from build123d import *

# Parameters (mm, degrees)
SALIENTE_EXTRUIR1_DEPTH = 5.75
CROQUIS2_W              = 25
CROQUIS2_H              = 25
SALIENTE_EXTRUIR2_DEPTH = 3
CROQUIS3_W              = 21.75
CROQUIS3_H              = 21.75
CROQUIS3_W_2            = 13.5
CROQUIS3_H_2            = 13.5
SALIENTE_EXTRUIR3_DEPTH = 13
CORTAR_EXTRUIR1_DEPTH   = 13
CORTAR_EXTRUIR2_DEPTH   = 13
SALIENTE_EXTRUIR4_DEPTH = 2


with BuildPart() as part:
    # Croquis1 → Saliente-Extruir1 (new, symmetric)
    with BuildSketch(Plane(origin=(0, 0, 0), x_dir=(1, 0, 0), z_dir=(0, 1, 0))):
        Polygon((0, 0), (15, 0), (15, -10), (-10, -10), (-10, 15), (0, 15), align=None)
    extrude(amount=SALIENTE_EXTRUIR1_DEPTH, both=True)

    # Croquis2 → Saliente-Extruir2 (add)
    with BuildSketch(Plane.XZ.offset(5.75)):
        with Locations((2.5, -2.5)):
            Rectangle(CROQUIS2_W, CROQUIS2_H)
    extrude(amount=SALIENTE_EXTRUIR2_DEPTH)

    # Croquis3 → Saliente-Extruir3 (add)
    with BuildSketch(Plane.XZ.offset(8.75)):
        with Locations((0.875, -0.875)):
            Rectangle(CROQUIS3_W, CROQUIS3_H)
        with Locations((2.5, -2.5)):
            Rectangle(CROQUIS3_W_2, CROQUIS3_H_2, mode=Mode.SUBTRACT)
    extrude(amount=SALIENTE_EXTRUIR3_DEPTH)

    # Croquis4 → Cortar-Extruir1 (cut)
    with BuildSketch(Plane(origin=(11.75, 0, 0), x_dir=(0, 0, -1), z_dir=(1, 0, 0))):
        with BuildLine():
            Line((-1.125, -12.25), (-1.125, -18.25))
            ThreePointArc((-1.125, -18.25), (0.875, -20.25), (2.875, -18.25))
            Line((2.875, -18.25), (2.875, -12.25))
            ThreePointArc((2.875, -12.25), (0.875, -10.25), (-1.125, -12.25))
        make_face()
    extrude(amount=-CORTAR_EXTRUIR1_DEPTH, mode=Mode.SUBTRACT)

    # Croquis6 → Cortar-Extruir2 (cut)
    with BuildSketch(Plane(origin=(0, 0, -11.75), x_dir=(-1, 0, 0), z_dir=(0, 0, -1))):
        with BuildLine():
            Line((1.125, -12.25), (1.125, -18.25))
            ThreePointArc((1.125, -18.25), (-0.875, -20.25), (-2.875, -18.25))
            Line((-2.875, -18.25), (-2.875, -12.25))
            ThreePointArc((-2.875, -12.25), (-0.875, -10.25), (1.125, -12.25))
        make_face()
    extrude(amount=-CORTAR_EXTRUIR2_DEPTH, mode=Mode.SUBTRACT)

    # Croquis7 → Saliente-Extruir4 (add)
    with BuildSketch(Plane(origin=(0, 5.75, 0), x_dir=(1, 0, 0), z_dir=(0, 1, 0))):
        Polygon((15, 0), (0, 15), (0, 0), align=None)
        Polygon((15, 0), (0, 0), (0, 15), (-10, 15), (-10, -10), (15, -10), align=None)
    extrude(amount=SALIENTE_EXTRUIR4_DEPTH)


solid = part.part
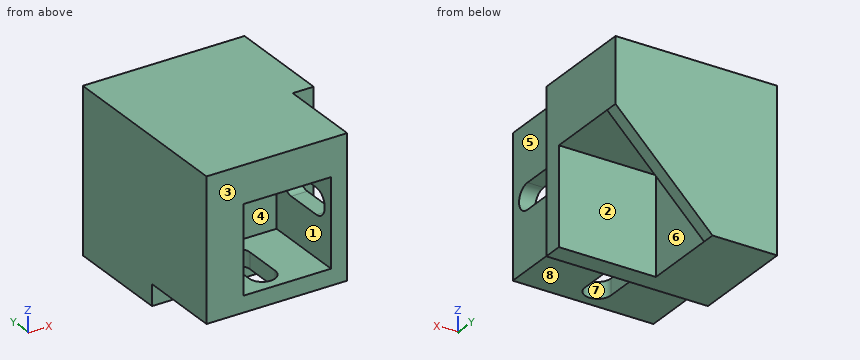
CAD build for the part. Positions are in the model's coordinates, mm. Face numbers are marked on the shaded views. A direction names the side the tool comes from. Coordinates: 2 decimals unless noted, no trailing zeros. Write each loop counter-clockwise with the first axis right and the second up, starting at its lowest first coordinate (ties: lowest second). Pieces come first, ordered by that corner, then holes. Notation, with made-up numbers: M 66.5,8 L 99.5,8 A25 ccw 99.5,27 Z; hole C 25,8 d10. An arc over 180 degrees is marked long. Return JSON: item names as keys, results as strings.
Item 1: Drop flat-ended pins along their axis: pin 1 Ø6.5 at (y, z) = (-12.5, -2) entering from +X; pin 2 Ø3 at (x, y) = (11, -14.5) entering from -Z; pin 3 Ø4 at (x, z) = (3.5, 0.5) entering from -Y. Give the stop position or say it passes through.
Findings below:
{"pin 1": "stops at x = 11.75", "pin 2": "stops at z = -11.75", "pin 3": "stops at y = -8.75"}
Item 2: Slice it at B-B, the plane y = -16.75. Write the cut outline in (x, z) (3 decimals).
Findings below:
{"outline": "M -10,-11.75 L -1.125,-11.75 L -1.125,-9.25 L -4.25,-9.25 L -4.25,4.25 L 9.25,4.25 L 9.25,1.125 L 11.75,1.125 L 11.75,10 L -10,10 Z; M 2.875,-11.75 L 11.75,-11.75 L 11.75,-2.875 L 9.25,-2.875 L 9.25,-9.25 L 2.875,-9.25 Z"}
Item 3: Which spindle directions (+Z, -Z, +X, -X, +Y, -Y) get a long thin tool onto all of the face, cutting with end or side? Do the marked faces 4, 5, 6, 7 and 8. Say none if no direction does.
Findings below:
{"face 4": "-Y", "face 5": "+Z, -Z, +X, -Y", "face 6": "-Z, +X", "face 7": "-Z", "face 8": "-Z, +X, -X, -Y"}
Item 4: Slice it at D-D, the plane z = -0.5. Write the cut outline in (x, y), and give its area (3 significant figures).
Findings below:
{"outline": "M -10,-21.75 L -4.25,-21.75 L -4.25,-8.75 L 9.25,-8.75 L 9.25,-10.29 L 11.75,-10.29 L 11.75,-8.75 L 15,-8.75 L 15,-5.75 L 0,-5.75 L 0,5.75 L 14.5,5.75 L 14.5,7.75 L -10,7.75 Z; M 9.25,-21.75 L 11.75,-21.75 L 11.75,-20.21 L 9.25,-20.21 Z", "area": "321 mm2"}
Item 5: Probe line 1 (X direction, y = -18.5, z = -4); line 2 (Y direction, x = 3.5, z = -2); line 3 (Z direction, x = 7.75, y = -16.75). List the from-to ranges inside material, lowest first. Write a range as from..to.
Findings below:
{"line 1": "x = -10..-4.25, 9.25..11.75", "line 2": "y = -8.75..-5.75, 5.75..7.75", "line 3": "z = -11.75..-9.25, 4.25..10"}
Item 6: Two-plate mould, pull along Y, no slides. Class the marked faces 1, 2 and 3: +Y half, -Y half, draft (parallel to the pull), parting line (faces both ways), or undercut.
Findings below:
{"face 1": "draft", "face 2": "undercut", "face 3": "-Y half"}
Item 7: Slice it at C-C, the plane x = -2. Write the cut outline in (y, z).
Findings below:
{"outline": "M -21.75,-11.75 L -8.75,-11.75 L -8.75,-15 L 7.75,-15 L 7.75,10 L -21.75,10 L -21.75,4.25 L -8.75,4.25 L -8.75,-9.25 L -21.75,-9.25 Z"}
Item 8: Slice it at A-A, the plane z = -4. Write the cut outline in (x, y).
Findings below:
{"outline": "M -10,-21.75 L -4.25,-21.75 L -4.25,-8.75 L 9.25,-8.75 L 9.25,-21.75 L 11.75,-21.75 L 11.75,-8.75 L 15,-8.75 L 15,-5.75 L 0,-5.75 L 0,5.75 L 11,5.75 L 11,7.75 L -10,7.75 Z"}
